Read the model definition and answer for the solid it produces. Units are mm, in the model's axes. A direction names the side the tool comes from. Coordinates: 2 decimals unless noted, no trailing zeros. Write each loop counter-clockwise with the first axis right and the second up, starting at its lowest first coordinate (ties: lowest second). Pieces come first, ordered by that corner, then holes. Notation, with made-up numbers: (18.25, 50.25) -> (77.25, 50.25) arc R35 ccw to (77.25, 86.25) -> close; hole circle Ø1 at (-10.5, 19.25). An arc over 180 degrees is marked (long way). Return JSON: item names as keys, results as strings.
from build123d import *

# Parameters (mm, degrees)
SKETCH1_R           = 5
BOSS_EXTRUDE1_DEPTH = 103
SKETCH5_W           = 1
SKETCH5_H           = 4


with BuildPart() as part:
    # Sketch1 → Boss-Extrude1 (new body)
    with BuildSketch(Plane(origin=(0, 0, 0), x_dir=(1, 0, 0), z_dir=(0, 1, 0))):
        Circle(SKETCH1_R)
    extrude(amount=BOSS_EXTRUDE1_DEPTH)

    # Sketch4 → Ø4.0mm Dowel Hole1 (revolve, cut)
    with BuildSketch(Plane(origin=(0, 103, 0), x_dir=(0, 0, 1), z_dir=(1, 0, 0))):
        Polygon((0, 0), (0, 19.201721238), (2, 18), (2, 0.025), (2.025, 0), align=None)
    f_4_0mm_dowel_hole1 = revolve(axis=Axis((0, 109.35, 0), (0, -1, 0)), mode=Mode.SUBTRACT)

    # Mirror1: Ø4.0mm Dowel Hole1 across plane
    add(f_4_0mm_dowel_hole1.mirror(Plane.ZX.offset(51.5)), mode=Mode.SUBTRACT)

    # Sketch5 → Cut-Revolve2 (revolve, cut)
    with BuildSketch(Plane.XY):
        with Locations((-4.5, 101)):
            Rectangle(SKETCH5_W, SKETCH5_H)
        with Locations((-4.5, 2)):
            Rectangle(SKETCH5_W, SKETCH5_H)
    revolve(axis=Axis((0, 103, 0), (0, -1, 0)), mode=Mode.SUBTRACT)


solid = part.part
1. The part is cut by section A-A (y = 91.5). Determine the outline of the cut face in (x, z).
Taken from the geometry:
{"outline": "circle Ø10 at (0, 0); hole circle Ø4 at (0, 0)"}
2. For a pull along X with two mould halves and no side action, classify faces 3 (the face through (2, 9, 0)), 4 (the face through (-2, 0, -1)), 5 (the face through (2, 94, 0)), 6 (the face through (0.867, 2.028, 3.905)) as +X half, -X half, draft (parallel to the pull), parting line (faces both ways), or undercut.
Taken from the geometry:
{"face 3": "undercut", "face 4": "draft", "face 5": "undercut", "face 6": "parting line"}
3. Consider L1, parallel to Z at x = 0, y = 14; L2, parallel to X at y = 15.5, z = -1; L3, parallel to X at y = 52, z = 3. Determine where each line is inside the solid, lowest interval first.
Taken from the geometry:
{"L1": "z = -5 to -2, 2 to 5", "L2": "x = -4.9 to -1.73, 1.73 to 4.9", "L3": "x = -4 to 4"}
4. A tool of negligible diameter and unlimited length cuts with its end or side. For faces 1 (the face through (-1.08, 50.84, 4.88)), 2 (the face through (0.867, 101.028, 3.905)), from which of +Z, -Z, +X, -X, +Y, -Y can it reach the whole face along a straight path? Write none if from no direction.
Taken from the geometry:
{"face 1": "+Y, -Y", "face 2": "+Y"}
5. The part is cut by section B-B (y = 23). Determine the outline of the cut face in (x, z).
Taken from the geometry:
{"outline": "circle Ø10 at (0, 0)"}
6. Flat-ended cylindrical pins translate along their axes: pin 1 Ø2 at (y, z) = (19.5, -2.5) entering from -X; pin 2 Ø1.5 at (y, z) = (71, 4) entering from +X; pin 3 Ø3.5 at (x, z) = (0, 0) entering from +Y. Find the tip coordinate at first contact, or state that the pin passes through.
Taken from the geometry:
{"pin 1": "stops at x = -4.77", "pin 2": "stops at x = 3.8", "pin 3": "stops at y = 84.85"}
